For this review, take the finished solid that the model builds, in its own axes (mm). A direction names the side the tool comes from. Round coordinates to 2 decimals unless told otherwise and drop trailing zeros. Write each loop counter-clockwise with the first axis right and the second up, starting at its lowest first coordinate (ties: lowest second). Pieces come first, ordered by that corner, then holes.
from build123d import *

# Parameters (mm, degrees)
SKETCH1_R           = 4
BOSS_EXTRUDE1_DEPTH = 15
BOSS_EXTRUDE2_START = 2
BOSS_EXTRUDE2_DEPTH = 2
SKETCH3_R           = 1.5
CUT_EXTRUDE1_DEPTH  = 49.692915296
FILLET1_R           = 8
CUT_EXTRUDE2_DEPTH  = 3


with BuildPart() as part:
    # Sketch1 → Boss-Extrude1 (new body)
    with BuildSketch(Plane.XY):
        with BuildLine():
            Line((-45, 0), (45, 0))
            Line((45, 0), (45, 11))
            Line((45, 11), (30, 11))
            ThreePointArc((30, 11), (25, 16), (20, 11))
            Line((20, 11), (20, 3))
            Line((20, 3), (-20, 3))
            Line((-20, 3), (-20, 11))
            ThreePointArc((-20, 11), (-25, 16), (-30, 11))
            Line((-30, 11), (-45, 11))
            Line((-45, 11), (-45, 0))
        make_face()
        with Locations((25, 11)):
            Circle(SKETCH1_R, mode=Mode.SUBTRACT)
        with Locations(Location((-25, 11, 0), (0, 0, 180))):
            Circle(SKETCH1_R, mode=Mode.SUBTRACT)
    extrude(amount=BOSS_EXTRUDE1_DEPTH)

    # Sketch2 → Boss-Extrude2 (add)
    with BuildSketch(Plane(origin=(0, 0, 0), x_dir=(-1, 0, 0), z_dir=(0, 0, -1)).offset(BOSS_EXTRUDE2_START)):
        with BuildLine():
            Line((-45, 11), (-45, 0))
            Line((-45, 0), (45, 0))
            Line((45, 0), (45, 11))
            Line((45, 11), (30, 11))
            ThreePointArc((30, 11), (25, 16), (20, 11))
            Line((20, 11), (20, 3))
            Line((20, 3), (-20, 3))
            Line((-20, 3), (-20, 11))
            ThreePointArc((-20, 11), (-25, 16), (-30, 11))
            Line((-30, 11), (-45, 11))
        make_face()
    extrude(amount=-BOSS_EXTRUDE2_DEPTH)

    # Sketch3 → Cut-Extrude1 (cut, through all)
    with BuildSketch(Plane(origin=(0, 11, 0), x_dir=(1, 0, 0), z_dir=(0, 1, 0))):
        with Locations(Location((38, -6.5, 0), (0, 0, 270))):
            Circle(SKETCH3_R)
    cut_extrude1 = extrude(amount=-CUT_EXTRUDE1_DEPTH, mode=Mode.SUBTRACT)

    # Mirror1: Cut-Extrude1 across plane
    add(cut_extrude1.mirror(Plane(origin=(0, 0, 0), x_dir=(0, 0, 1), z_dir=(1, 0, 0))), mode=Mode.SUBTRACT)

    # Fillet1
    fillet1_edges = [part.edges().sort_by_distance(p)[0] for p in [
        (-45, 5.5, 15),
        (45, 5.5, 15),
        (45, 5.5, -2),
        (-45, 5.5, -2),
    ]]
    fillet(fillet1_edges, radius=FILLET1_R)

    # Sketch4 → Cut-Extrude2 (cut)
    with BuildSketch(Plane(origin=(0, 11, 0), x_dir=(1, 0, 0), z_dir=(0, 1, 0))):
        Polygon((38, -3.035898385), (35, -4.767949192), (35, -8.232050808), (38, -9.964101615), (41, -8.232050808), (41, -4.767949192), align=None)
    cut_extrude2 = extrude(amount=-CUT_EXTRUDE2_DEPTH, mode=Mode.SUBTRACT)

    # Mirror3: Cut-Extrude2 across plane
    add(cut_extrude2.mirror(Plane(origin=(0, 0, 0), x_dir=(0, 0, 1), z_dir=(1, 0, 0))), mode=Mode.SUBTRACT)


solid = part.part
(1) For line 1 along X through (y, z) = (2, 6.5); line 2 along X through (y, z) = (6, 6.5); line 3 along Y through (x, z) = (-25, 10.25), list the stretches that pass through material, from the lowest coordinate up.
Geometry check:
line 1: x = -45 to -39.5, -36.5 to 36.5, 39.5 to 45
line 2: x = -45 to -39.5, -36.5 to -20, 20 to 36.5, 39.5 to 45
line 3: y = 0 to 7, 15 to 16
(2) We need section D-D, the plane y = 12. Give the boundary of the cut face in (x, z), and give its area (3 significant figures).
Geometry check:
outline: (-29.9, -2) - (-20.1, -2) - (-20.1, 15) - (-21.13, 15) - (-21.13, 0) - (-28.87, 0) - (-28.87, 15) - (-29.9, 15) - close; (20.1, -2) - (29.9, -2) - (29.9, 15) - (28.87, 15) - (28.87, 0) - (21.13, 0) - (21.13, 15) - (20.1, 15) - close
area: 101 mm2
(3) We need section B-B, the plane z = 10.75. Give the boundary of the cut face in (x, y).
Geometry check:
outline: (-44.07, 0) - (44.07, 0) - (44.07, 11) - (30, 11) arc R5 ccw to (20, 11) - (20, 3) - (-20, 3) - (-20, 11) arc R5 ccw to (-30, 11) - (-44.07, 11) - close; hole circle Ø8 at (-25, 11); hole circle Ø8 at (25, 11)
(4) Mouldability with a two-part tool opening along Z and no side actions: class faces 6 (the face through (42.719, 5.423, 0.406)), 7 (the face through (-36.536, 4.056, 6.175)), 8 (the face through (-21.8, 13.4, 7.4)) as pulls with the +Z half, pulls with the -Z half, needs draft (parallel to the pull), parting line crosses it, or undercut.
Geometry check:
face 6: pulls with the -Z half
face 7: undercut
face 8: needs draft
(5) For pin 1 Ø6.5 at (y, z) = (7.5, 2.5) entering from +X; pin 2 Ø7.5 at (x, z) = (-36, 9.5) entering from +Y; pin 3 Ø1.8 at (x, z) = (37, 6) entering from +Y, all flat-tipped, find the tip position at first contact; note any pin that passes through.
Geometry check:
pin 1: stops at x = 45
pin 2: stops at y = 11
pin 3: stops at y = 8
(6) We need section A-A, the plane y = 5.25. Give the boundary of the cut face in (x, z).
Geometry check:
outline: (-45, 6) arc R8 ccw to (-37, -2) - (-20, -2) - (-20, 15) - (-37, 15) arc R8 ccw to (-45, 7) - close; (20, -2) - (37, -2) arc R8 ccw to (45, 6) - (45, 7) arc R8 ccw to (37, 15) - (20, 15) - close; hole circle Ø3 at (-38, 6.5); hole circle Ø3 at (38, 6.5)
(7) We need section C-C, the plane x = -23.5. Give the boundary of the cut face in (y, z), and give its area (3 significant figures).
Geometry check:
outline: (0, -2) - (15.77, -2) - (15.77, 15) - (14.71, 15) - (14.71, 0) - (7.29, 0) - (7.29, 15) - (0, 15) - close
area: 157 mm2
(8) For faces 1 (the face through (20, 7, 6)), 2 (the face through (34, 11, 6)), 3 (the face through (-41, 10, 7)), 4 (the face through (-34, 11, 6)), 5 (the face through (1, 0, 6)), list the 3-axis set-ups (+Z, -Z, +X, -X, +Y, -Y) from which the entire face can be reached by the end or side of a thin tool; tool diameter is ignored.
Geometry check:
face 1: +Z, -Z, +Y
face 2: +Z, -Z, +X, +Y
face 3: +Y
face 4: +Z, -Z, -X, +Y
face 5: +Z, -Z, +X, -X, -Y
